```python
from build123d import *

# Parameters (mm, degrees)
SKETCH_1_W                        = 628
SKETCH_1_H                        = 348
SM_BASE_FLANGE_1_DEPTH            = 2
SM_EDGE_FLANGE_1_STRIP_W          = 9
SM_EDGE_FLANGE_1_STRIP_H          = 2
SM_EDGE_FLANGE_1_STRIP_CUT_DEPTH  = 248
SM_EDGE_FLANGE_1_RELIEF_W         = 10
SM_EDGE_FLANGE_1_RELIEF_H         = 1
SM_EDGE_FLANGE_1_RELIEF_CUT_DEPTH = 2
SM_EDGE_FLANGE_1_DEPTH            = 248
SM_EDGE_FLANGE_2_STRIP_W          = 9
SM_EDGE_FLANGE_2_STRIP_H          = 2
SM_EDGE_FLANGE_2_STRIP_CUT_DEPTH  = 528
SM_EDGE_FLANGE_2_RELIEF_W         = 10
SM_EDGE_FLANGE_2_RELIEF_H         = 1
SM_EDGE_FLANGE_2_RELIEF_CUT_DEPTH = 2
SM_EDGE_FLANGE_2_DEPTH            = 528
SM_EDGE_FLANGE_2_FLAT_DEPTH       = 2
SM_EDGE_FLANGE_3_STRIP_W          = 9
SM_EDGE_FLANGE_3_STRIP_H          = 2
SM_EDGE_FLANGE_3_STRIP_CUT_DEPTH  = 248
SM_EDGE_FLANGE_3_RELIEF_W         = 10
SM_EDGE_FLANGE_3_RELIEF_H         = 1
SM_EDGE_FLANGE_3_RELIEF_CUT_DEPTH = 2
SM_EDGE_FLANGE_3_DEPTH            = 248
SM_EDGE_FLANGE_4_STRIP_W          = 9
SM_EDGE_FLANGE_4_STRIP_H          = 2
SM_EDGE_FLANGE_4_STRIP_CUT_DEPTH  = 528
SM_EDGE_FLANGE_4_RELIEF_W         = 10
SM_EDGE_FLANGE_4_RELIEF_H         = 1
SM_EDGE_FLANGE_4_RELIEF_CUT_DEPTH = 2
SM_EDGE_FLANGE_4_DEPTH            = 528
SKETCH_15_R                       = 3.5
CUT_EXTRUDE_1_DEPTH               = 653.030674125
CUT_EXTRUDE_2_REACH               = 469.756
SKETCH_16_R                       = 3.5
HOLE_WIZARD_M6_1_D                = 5
HOLE_WIZARD_M6_1_DEPTH            = 15
HOLE_WIZARD_M6_1_TIP              = 1.502151548
CUT_EXTRUDE_3_REACH               = 471.238
SKETCH_20_R                       = 3.5


# Sheet-metal steps are written as plain solids
with BuildPart() as part:
    # Sketch 1 → 基体-法兰1 (new body)
    with BuildSketch(Plane.XY):
        Rectangle(SKETCH_1_W, SKETCH_1_H)
    extrude(amount=-SM_BASE_FLANGE_1_DEPTH)

    # 边线-法兰1 strip (across the edge) → 边线-法兰1 strip cut (cut)
    with BuildSketch(Plane(origin=(314, 124, -2), x_dir=(-1, 0, 0), z_dir=(0, -1, 0))):
        with Locations((-2, -1)):
            Rectangle(SM_EDGE_FLANGE_1_STRIP_W, SM_EDGE_FLANGE_1_STRIP_H)
    extrude(amount=SM_EDGE_FLANGE_1_STRIP_CUT_DEPTH, mode=Mode.SUBTRACT)

    # 边线-法兰1 relief (on the sheet) → 边线-法兰1 relief cut (cut)
    with BuildSketch(Plane(origin=(311.5, 124, -2), x_dir=(-1, 0, 0), z_dir=(0, 0, -1))):
        with Locations((-4, 0.5)):
            Rectangle(SM_EDGE_FLANGE_1_RELIEF_W, SM_EDGE_FLANGE_1_RELIEF_H)
        with Locations((-4, -248.5)):
            Rectangle(SM_EDGE_FLANGE_1_RELIEF_W, SM_EDGE_FLANGE_1_RELIEF_H)
    extrude(amount=-SM_EDGE_FLANGE_1_RELIEF_CUT_DEPTH, mode=Mode.SUBTRACT)

    # 边线-法兰1 section (across the edge) → 边线-法兰1 (add)
    with BuildSketch(Plane(origin=(314, 124, -2), x_dir=(-1, 0, 0), z_dir=(0, -1, 0))):
        with BuildLine():
            Line((0, 0.5), (0, 20))
            Line((0, 20), (2, 20))
            Line((2, 20), (2, 0.5))
            ThreePointArc((2, 0.5), (2.146446609, 0.146446609), (2.5, 0))
            Line((2.5, 0), (2.5, -2))
            ThreePointArc((2.5, -2), (0.732233047, -1.267766953), (0, 0.5))
        make_face()
    extrude(amount=SM_EDGE_FLANGE_1_DEPTH)

    # 边线-法兰2 strip (across the edge) → 边线-法兰2 strip cut (cut)
    with BuildSketch(Plane(origin=(-264, 174, -2), x_dir=(0, -1, 0), z_dir=(1, 0, 0))):
        with Locations((-2, -1)):
            Rectangle(SM_EDGE_FLANGE_2_STRIP_W, SM_EDGE_FLANGE_2_STRIP_H)
    extrude(amount=SM_EDGE_FLANGE_2_STRIP_CUT_DEPTH, mode=Mode.SUBTRACT)

    # 边线-法兰2 relief (on the sheet) → 边线-法兰2 relief cut (cut)
    with BuildSketch(Plane(origin=(-264, 171.5, -2), x_dir=(0, -1, 0), z_dir=(0, 0, -1))):
        with Locations((-4, 0.5)):
            Rectangle(SM_EDGE_FLANGE_2_RELIEF_W, SM_EDGE_FLANGE_2_RELIEF_H)
        with Locations((-4, -528.5)):
            Rectangle(SM_EDGE_FLANGE_2_RELIEF_W, SM_EDGE_FLANGE_2_RELIEF_H)
    extrude(amount=-SM_EDGE_FLANGE_2_RELIEF_CUT_DEPTH, mode=Mode.SUBTRACT)

    # 边线-法兰2 bend section (across the edge) → 边线-法兰2 (add)
    with BuildSketch(Plane(origin=(-264, 174, -2), x_dir=(0, -1, 0), z_dir=(1, 0, 0))):
        with BuildLine():
            Line((0, 0.5), (2, 0.5))
            ThreePointArc((2, 0.5), (2.146446609, 0.146446609), (2.5, 0))
            Line((2.5, 0), (2.5, -2))
            ThreePointArc((2.5, -2), (0.732233047, -1.267766953), (0, 0.5))
        make_face()
    extrude(amount=SM_EDGE_FLANGE_2_DEPTH)

    # 边线-法兰2 profile (on flange) → 边线-法兰2 flat (add)
    with BuildSketch(Plane(origin=(0, 174, -2), x_dir=(1, 0, 0), z_dir=(0, 1, 0))):
        Polygon((264, 0.5), (264, 10), (-23, 10), (-23, 20), (-47, 20), (-47, 10), (-264, 10), (-264, 0.5), align=None)
    extrude(amount=-SM_EDGE_FLANGE_2_FLAT_DEPTH)

    # 边线-法兰3 strip (across the edge) → 边线-法兰3 strip cut (cut)
    with BuildSketch(Plane(origin=(-314, -124, -2), x_dir=(1, 0, 0), z_dir=(0, 1, 0))):
        with Locations((-2, -1)):
            Rectangle(SM_EDGE_FLANGE_3_STRIP_W, SM_EDGE_FLANGE_3_STRIP_H)
    extrude(amount=SM_EDGE_FLANGE_3_STRIP_CUT_DEPTH, mode=Mode.SUBTRACT)

    # 边线-法兰3 relief (on the sheet) → 边线-法兰3 relief cut (cut)
    with BuildSketch(Plane(origin=(-311.5, -124, -2), x_dir=(1, 0, 0), z_dir=(0, 0, -1))):
        with Locations((-4, 0.5)):
            Rectangle(SM_EDGE_FLANGE_3_RELIEF_W, SM_EDGE_FLANGE_3_RELIEF_H)
        with Locations((-4, -248.5)):
            Rectangle(SM_EDGE_FLANGE_3_RELIEF_W, SM_EDGE_FLANGE_3_RELIEF_H)
    extrude(amount=-SM_EDGE_FLANGE_3_RELIEF_CUT_DEPTH, mode=Mode.SUBTRACT)

    # 边线-法兰3 section (across the edge) → 边线-法兰3 (add)
    with BuildSketch(Plane(origin=(-314, -124, -2), x_dir=(1, 0, 0), z_dir=(0, 1, 0))):
        with BuildLine():
            Line((0, 0.5), (0, 20))
            Line((0, 20), (2, 20))
            Line((2, 20), (2, 0.5))
            ThreePointArc((2, 0.5), (2.146446609, 0.146446609), (2.5, 0))
            Line((2.5, 0), (2.5, -2))
            ThreePointArc((2.5, -2), (0.732233047, -1.267766953), (0, 0.5))
        make_face()
    extrude(amount=SM_EDGE_FLANGE_3_DEPTH)

    # 边线-法兰4 strip (across the edge) → 边线-法兰4 strip cut (cut)
    with BuildSketch(Plane(origin=(264, -174, -2), x_dir=(0, 1, 0), z_dir=(-1, 0, 0))):
        with Locations((-2, -1)):
            Rectangle(SM_EDGE_FLANGE_4_STRIP_W, SM_EDGE_FLANGE_4_STRIP_H)
    extrude(amount=SM_EDGE_FLANGE_4_STRIP_CUT_DEPTH, mode=Mode.SUBTRACT)

    # 边线-法兰4 relief (on the sheet) → 边线-法兰4 relief cut (cut)
    with BuildSketch(Plane(origin=(264, -171.5, -2), x_dir=(0, 1, 0), z_dir=(0, 0, -1))):
        with Locations((-4, 0.5)):
            Rectangle(SM_EDGE_FLANGE_4_RELIEF_W, SM_EDGE_FLANGE_4_RELIEF_H)
        with Locations((-4, -528.5)):
            Rectangle(SM_EDGE_FLANGE_4_RELIEF_W, SM_EDGE_FLANGE_4_RELIEF_H)
    extrude(amount=-SM_EDGE_FLANGE_4_RELIEF_CUT_DEPTH, mode=Mode.SUBTRACT)

    # 边线-法兰4 section (across the edge) → 边线-法兰4 (add)
    with BuildSketch(Plane(origin=(264, -174, -2), x_dir=(0, 1, 0), z_dir=(-1, 0, 0))):
        with BuildLine():
            Line((0, 0.5), (0, 20))
            Line((0, 20), (2, 20))
            Line((2, 20), (2, 0.5))
            ThreePointArc((2, 0.5), (2.146446609, 0.146446609), (2.5, 0))
            Line((2.5, 0), (2.5, -2))
            ThreePointArc((2.5, -2), (0.732233047, -1.267766953), (0, 0.5))
        make_face()
    extrude(amount=SM_EDGE_FLANGE_4_DEPTH)

    # 草图15 → 切除-拉伸1 (cut, through all)
    with BuildSketch(Plane(origin=(314, 0, 0), x_dir=(0, 0, -1), z_dir=(1, 0, 0))):
        with Locations((12, -105)):
            Circle(SKETCH_15_R)
        with Locations((12, 105)):
            Circle(SKETCH_15_R)
    extrude(amount=-CUT_EXTRUDE_1_DEPTH, mode=Mode.SUBTRACT)

    # 草图16 → 切除-拉伸2 (cut, up to next)
    with BuildSketch(Plane.XZ.offset(-172), mode=Mode.PRIVATE) as cut_extrude_2_sk1:
        with Locations(Location((-35, -12, 0), (0, 0, 270))):
            Circle(SKETCH_16_R)
    cut_extrude_2_tool1 = extrude(cut_extrude_2_sk1.sketch, amount=-CUT_EXTRUDE_2_REACH, mode=Mode.PRIVATE) & part.part
    add(cut_extrude_2_tool1.solids().sort_by_distance((-35, 172, -12))[0], mode=Mode.SUBTRACT)

    # M6 螺纹孔1
    with Locations(Plane(origin=(0, 0, -2), x_dir=(-1, 0, 0), z_dir=(0, 0, -1))):
        with Locations((-194.6, 71.5), (-54.6, 71.5), (-54.6, -108.5), (-194.6, -108.5)):
            Hole(HOLE_WIZARD_M6_1_D / 2, depth=HOLE_WIZARD_M6_1_DEPTH)
            with Locations((0, 0, -(HOLE_WIZARD_M6_1_DEPTH + HOLE_WIZARD_M6_1_TIP / 2))):  # 118° drill point
                Cone(0, HOLE_WIZARD_M6_1_D / 2, HOLE_WIZARD_M6_1_TIP, mode=Mode.SUBTRACT)

    # 草图20 → 切除-拉伸3 (cut, up to next)
    with BuildSketch(Plane.XZ.offset(174), mode=Mode.PRIVATE) as cut_extrude_3_sk1:
        with Locations(Location((0, -12, 0), (0, 0, 270))):
            Circle(SKETCH_20_R)
    cut_extrude_3_tool1 = extrude(cut_extrude_3_sk1.sketch, amount=-CUT_EXTRUDE_3_REACH, mode=Mode.PRIVATE) & part.part
    # 草图20 → 切除-拉伸3 (cut, up to next)
    with BuildSketch(Plane.XZ.offset(174), mode=Mode.PRIVATE) as cut_extrude_3_sk2:
        with Locations(Location((-250, -12, 0), (0, 0, 270))):
            Circle(SKETCH_20_R)
    cut_extrude_3_tool2 = extrude(cut_extrude_3_sk2.sketch, amount=-CUT_EXTRUDE_3_REACH, mode=Mode.PRIVATE) & part.part
    # 草图20 → 切除-拉伸3 (cut, up to next)
    with BuildSketch(Plane.XZ.offset(174), mode=Mode.PRIVATE) as cut_extrude_3_sk3:
        with Locations(Location((250, -12, 0), (0, 0, 270))):
            Circle(SKETCH_20_R)
    cut_extrude_3_tool3 = extrude(cut_extrude_3_sk3.sketch, amount=-CUT_EXTRUDE_3_REACH, mode=Mode.PRIVATE) & part.part
    add(cut_extrude_3_tool1.solids().sort_by_distance((0, -174, -12))[0], mode=Mode.SUBTRACT)
    add(cut_extrude_3_tool2.solids().sort_by_distance((-250, -174, -12))[0], mode=Mode.SUBTRACT)
    add(cut_extrude_3_tool3.solids().sort_by_distance((250, -174, -12))[0], mode=Mode.SUBTRACT)


solid = part.part
```
Check sheet for the modelled part. Datum: model origin and axes. Units: mm. A direction names the side the tool comes from. Coordinates: 2 decimals unless noted, no trailing zeros. Write each loop counter-clockwise with the first axis right and the second up, starting at its lowest first coordinate (ties: lowest second). Pieces come first, ordered by that corner, then holes. Notation, with made-up numbers: M 12.25,25 L 45.25,25 A10 cw 45.25,37 Z; hole C -33.75,15.25 d9. An arc over 180 degrees is marked long. Use one line per item in the form item = value.
Item 1: Material ranges on L1, parallel to X at y = -173.15, z = -12; L2, parallel to Y at x = 54.6, z = -1.05; L3, parallel to Y at x = 313.15, z = -12, recorded low to high. Write a range as from..to.
Answer below:
L1 = -264..-253.5, -246.5..-3.5, 3.5..246.5, 253.5..264
L2 = -173.54..-111, -106..69, 74..173.54
L3 = -124..-108.5, -101.5..101.5, 108.5..124
Item 2: Sectioned sample at B-B, the plane x = 149. Record the cut outline in (y, z), and give its area (3 significant figures).
Answer below:
outline = M -174,-22 L -172,-22 L -172,-2.5 A0.5 cw -171.5,-2 L 171.5,-2 A0.5 cw 172,-2.5 L 172,-12 L 174,-12 L 174,-2.5 A2.5 ccw 171.5,0 L -171.5,0 A2.5 ccw -174,-2.5 Z
area = 753 mm^2
Item 3: Gauge pin test, flat ends, axial feed: pin 1 Ø0.6 at (y, z) = (173, -14.5) entering from +X; pin 2 Ø6 at (x, y) = (-199.5, -6) entering from -Z; pin 3 Ø4 at (y, z) = (105, -12) entering from +X; pin 4 Ø0.5 at (y, z) = (124.5, -1) entering from +X. Record the tip position at first contact, or that the pin passes through.
Answer below:
pin_1 = -23
pin_2 = -2
pin_3 = through
pin_4 = 310.5
Item 4: Set-up check for faces 5 (the face through (-4, 2, -2)), 6 (the face through (-4, 172, -8)), 7 (the face through (312, 2, -12)): record each of +Z, -Z, +X, -X, +Y, -Y from which the full face is reachable in a straight line by a thin tool's end or side.
Answer below:
face_5 = -Z
face_6 = -Z, +X, -X
face_7 = -Z, +Y, -Y
Item 5: Sectioned sample at A-A, the plane y = 0. Record the cut outline in (x, z).
Answer below:
outline = M -314,-22 L -312,-22 L -312,-2.5 A0.5 cw -311.5,-2 L 311.5,-2 A0.5 cw 312,-2.5 L 312,-22 L 314,-22 L 314,-2.5 A2.5 ccw 311.5,0 L -311.5,0 A2.5 ccw -314,-2.5 Z
Item 6: Release check for a two-part mould opening along Y. For faces 1 (the face through (-4, 174, -8)), 2 (the face through (4, -172, -12)), 3 (the face through (-312, -2, -12)), 4 (the face through (4, -174, -12)) record: pulls with the +Y half, pulls with the -Y half, needs draft (parallel to the pull), parting line crosses it, or undercut.
Answer below:
face_1 = pulls with the +Y half
face_2 = undercut
face_3 = needs draft
face_4 = pulls with the -Y half
